```python
from build123d import *

# Parameters (mm, degrees)
SKETCH1_R           = 25.4
SKETCH1_R_2         = 19.05
BOSS_EXTRUDE1_DEPTH = 25.4
SKETCH2_W           = 15.24
SKETCH2_H           = 6.35
SKETCH2_W_2         = 6.35
SKETCH2_H_2         = 15.24
CUT_EXTRUDE1_DEPTH  = 6.35
SKETCH3_W           = 19.80573375
SKETCH3_H           = 5.715
CUT_EXTRUDE2_DEPTH  = 2.667


with BuildPart() as part:
    # Sketch1 → Boss-Extrude1 (new body)
    with BuildSketch(Plane(origin=(0, 0, 0), x_dir=(1, 0, 0), z_dir=(0, 1, 0))):
        with Locations(Location((0, 0, 0), (0, 0, 270))):
            Circle(SKETCH1_R)
        with Locations(Location((0, 0, 0), (0, 0, 270))):
            Circle(SKETCH1_R_2, mode=Mode.SUBTRACT)
    extrude(amount=BOSS_EXTRUDE1_DEPTH)

    # Sketch2 → Cut-Extrude1 (cut)
    with BuildSketch(Plane.XZ):
        with Locations((25.4, 0)):
            Rectangle(SKETCH2_W, SKETCH2_H)
        with Locations((0, 25.4)):
            Rectangle(SKETCH2_W_2, SKETCH2_H_2)
    extrude(amount=-CUT_EXTRUDE1_DEPTH, mode=Mode.SUBTRACT)

    # Sketch3 → Cut-Extrude2 (cut)
    with BuildSketch(Plane(origin=(0, 25.4, 0), x_dir=(1, 0, 0), z_dir=(0, 1, 0))):
        with Locations((25.4, 0)):
            Rectangle(SKETCH3_W, SKETCH3_H)
    extrude(amount=-CUT_EXTRUDE2_DEPTH, mode=Mode.SUBTRACT)


solid = part.part
```
Part model, mm, in its own coordinate system. A direction names the side the tool comes from. Coordinates: 2 decimals unless noted, no trailing zeros. Write each loop counter-clockwise with the first axis right and the second up, starting at its lowest first coordinate (ties: lowest second). Pieces come first, ordered by that corner, then holes.
Item 1: Which spindle directions (+Z, -Z, +X, -X, +Y, -Y) get a long thin tool onto all of the face, cutting with end or side? Do faces 4 (the face through (3.175, 3, 22)), 5 (the face through (-18.597, 12.522, -4.13)), 6 (the face through (22, 3, 3.175)), 7 (the face through (22, 24, 2.858)). Say none if no direction does.
Item 2: Slice it at B-B (x = 0). Write the cut outline in (y, z), and give its area (3 significant figures).
Item 3: Slice it at D-D (y = 23.75). Write the cut outline in (x, z), and give its area (3 significant figures).
Item 4: Probe line 1 (X direction, y = 19.5, z = 0); line 2 (X direction, y = 11.5, z = -7.5). List the from-to ranges inside material, lowest first.
Item 5: Slice it at A-A (y = 3.25). Write the cut outline in (x, z) (3 decimals).
Item 6: Pin check, flat tips, straight feed: pin 1 (7 mm diameter, centred on y = 2.5, z = 22.5, fed in from -X); pin 2 (3 mm diameter, centred on x = 21, z = -1, fed in from +Y); pin 3 (5 mm diameter, centred on x = 22.5, z = -0.5, fed in from -Y); pin 4 (2 mm diameter, centred on x = 0.5, y = 10, fed in from -Z). Stop position of each tip, or through.
Item 7: Slice it at C-C (y = 9). Write the cut outline in (x, z), and give its area (3 significant figures).
Item 8: Mould opens along X. For faces 1 (the face through (-9, 0, -17)), 2 (the face through (0, 6.35, 22)), 3 (the face through (-15.456, 12.522, -20.157)) say: released by +X, released by -X, zero draft, split by the parting line, or undercut.
Results found:
1. face 4: +Z, -Y
1. face 5: +Y, -Y
1. face 6: +X, -Y
1. face 7: +X, +Y
2. outline: (0, -25.4) - (25.4, -25.4) - (25.4, -19.05) - (0, -19.05) - close; (6.35, 19.05) - (25.4, 19.05) - (25.4, 25.4) - (6.35, 25.4) - close
2. area: 282 mm2
3. outline: (18.83, -2.86) arc R19.05 cw (long way) to (18.83, 2.86) - (25.24, 2.86) arc R25.4 ccw (long way) to (25.24, -2.86) - close
3. area: 850 mm2
4. line 1: x = -25.4 to -19.05, 19.05 to 25.4
4. line 2: x = -24.27 to -17.51, 17.51 to 24.27
5. outline: (-3.175, 18.784) - (-3.175, 25.201) arc R25.4 ccw (long way) to (25.201, -3.175) - (18.784, -3.175) arc R19.05 cw (long way) to start; (3.175, 18.784) arc R19.05 cw to (18.784, 3.175) - (25.201, 3.175) arc R25.4 ccw to (3.175, 25.201) - close
6. pin 1: stops at x = -16.86
6. pin 2: stops at y = 22.73
6. pin 3: stops at y = 6.35
6. pin 4: stops at z = -25.4
7. outline: circle Ø50.8 at (0, 0); hole circle Ø38.1 at (0, 0)
7. area: 887 mm2
8. face 1: zero draft
8. face 2: undercut
8. face 3: split by the parting line
